Autodesk Inventor part; units mm, degrees
ref_plane "YZ Plane" through (0, 0, 0) normal (1, 0, 0) x (0, 1, 0)
ref_plane "XZ Plane" through (0, 0, 0) normal (0, 1, 0) x (-1, 0, 0)
ref_plane "XY Plane" through (0, 0, 0) normal (0, 0, 1) x (1, 0, 0)
sketch "스케치1" plane through (0, 0, 0) normal (0, 1, 0) x (-1, 0, 0)
  line L0 (-30, 30) -> (30, 30)
  line L1 (30, 30) -> (30, -30)
  line L2 (30, -30) -> (-30, -30)
  line L3 (-30, -30) -> (-30, 30)
  line L4 (-30, 30) -> (30, -30) construction
  line L5 (30, 30) -> (-30, -30) construction
  line L6 (-32.4, 32.4) -> (32.4, 32.4)
  line L7 (32.4, 32.4) -> (32.4, -32.4)
  line L8 (32.4, -32.4) -> (-32.4, -32.4)
  line L9 (-32.4, -32.4) -> (-32.4, 32.4)
  line L10 (-32.4, 32.4) -> (32.4, -32.4) construction
  line L11 (32.4, 32.4) -> (-32.4, -32.4) construction
  point P0 (0, 0)
  dimension "d45" = 60
  dimension "d46" = 60
  dimension "d47" = 2.4
extrude "돌출7" add sketch "스케치1" along normal blind 5 contours L0 L1 L2 L3 | L6 L7 L8 L9
sketch "스케치7" plane through (0, 5, 0) normal (0, 1, 0) x (1, 0, 0)
  line L0 (-30, -30) -> (30, -30)
  line L1 (30, -30) -> (30, 30)
  line L2 (30, 30) -> (-30, 30)
  line L3 (-30, 30) -> (-30, -30)
  line L4 (-30, -30) -> (30, 30) construction
  line L5 (30, -30) -> (-30, 30) construction
  line L6 (31.6, -31.6) -> (-31.6, -31.6)
  line L7 (-31.6, -31.6) -> (-31.6, 31.6)
  line L8 (-31.6, 31.6) -> (31.6, 31.6)
  line L9 (31.6, 31.6) -> (31.6, -31.6)
  line L10 (31.6, -31.6) -> (-31.6, 31.6) construction
  line L11 (-31.6, -31.6) -> (31.6, 31.6) construction
  point P0 (0, 0)
  dimension "d50" = 60
  dimension "d51" = 60
  dimension "d52" = 1.6
extrude "돌출8" cut sketch "스케치7" against normal blind 1.6
sketch "스케치8" plane through (0, 0, 0) normal (0, -1, 0) x (1, 0, 0)
  line L0 (-20, -2.5) -> (-10, -2.5)
  line L1 (-10, -2.5) -> (-10, 2.5)
  line L2 (-10, 2.5) -> (-20, 2.5)
  line L3 (-20, 2.5) -> (-20, -2.5)
  line L4 (-20, -2.5) -> (-10, 2.5) construction
  line L5 (-10, -2.5) -> (-20, 2.5) construction
  line L6 (10, -2.5) -> (20, -2.5)
  line L7 (20, -2.5) -> (20, 2.5)
  line L8 (20, 2.5) -> (10, 2.5)
  line L9 (10, 2.5) -> (10, -2.5)
  line L10 (10, -2.5) -> (20, 2.5) construction
  line L11 (20, -2.5) -> (10, 2.5) construction
  line L12 (32.4, 32.4) -> (32.4, -32.4)
  line L13 (32.4, 0) -> (20, 0)
  line L14 (-20, 0) -> (-32.4, 0)
  line L15 (-32.4, -32.4) -> (-32.4, 32.4)
  point P0 (0, 0)
  point P1 (-15, 0)
  point P2 (15, 0)
  dimension "d55" = 10
  dimension "d56" = 5
  dimension "d57" = 20
  dimension "d58" = 10
  dimension "d61" = 12.4
extrude "돌출9" add sketch "스케치8" along normal blind 10
sketch "스케치9" plane through (-10, 0, -2.5) normal (0, 0, -1) x (-1, 0, 0)
  line L0 (10, -10) -> (0, -10)
  circle A0 centre (5, -10) radius 5
  line L1 (-20, -10) -> (-30, -10)
  circle A1 centre (-25, -10) radius 5
  point P0 (-10, 0)
  dimension "d64" = 10
  dimension "d65" = 10
extrude "돌출10" add sketch "스케치9" against normal blind 5
sketch "스케치10" plane through (-10, 0, -2.5) normal (0, 0, -1) x (-1, 0, 0)
  arc A0 (0, -10) -> (10, -10) centre (5, -10) ccw
  circle A1 centre (5, -10) radius 1.25
  arc A2 (-30, -10) -> (-20, -10) centre (-25, -10) ccw
  circle A3 centre (-25, -10) radius 1.25
  point P0 (-10, 0)
  dimension "d68" = 2.5
  dimension "d69" = 2.5
extrude "돌출11" cut sketch "스케치10" against normal blind 5
sketch "스케치11" plane through (0, 0, 0) normal (0, -1, 0) x (1, 0, 0)
  circle A0 centre (0, 19.821) radius 1.25
  line L0 (-20, 2.5) -> (-10, 2.5)
  point P0 (0, 0)
  dimension "d72" = 2.5
  dimension "d73" = 17.321
extrude "돌출12" cut sketch "스케치11" against normal blind 5
properties part number "사각형 OV-PAM 5패턴 상단"
The model under review builds one solid part; all positions refer to its coordinate system, in mm. A direction names the side the tool comes from. Round coordinates to 2 decimals unless told otherwise and drop trailing zeros. Loops run counter-clockwise (first coordinate to the right, second up) from the corner with the lowest first, then second, coordinate; pieces in that order, holes last. Notation, with made-up numbers: M 76.25,39 L 109.25,39 A22 ccw 109.25,57 Z; hole C -32,-18 d11. An arc over 180 degrees is marked long. Write item = value, one per line.
Item 1: Take a section at B-B on z = 1.5. Write out the cut boundary in (x, y).
Return value:
outline = M -32.4,0 L -20,0 L -20,-10 A5 ccw -10,-10 L -10,0 L 10,0 L 10,-10 A5 ccw 20,-10 L 20,0 L 32.4,0 L 32.4,5 L 31.6,5 L 31.6,3.4 L 30,3.4 L 30,5 L -30,5 L -30,3.4 L -31.6,3.4 L -31.6,5 L -32.4,5 Z; hole C -15,-10 d2.5; hole C 15,-10 d2.5
Item 2: Take a section at D-D on x = 9. Write out the cut boundary in (y, z).
Return value:
outline = M 0,-32.4 L 5,-32.4 L 5,-31.6 L 3.4,-31.6 L 3.4,-30 L 5,-30 L 5,30 L 3.4,30 L 3.4,31.6 L 5,31.6 L 5,32.4 L 0,32.4 Z
Item 3: Take a section at C-C on x = -15. Write out the cut boundary in (y, z).
Return value:
outline = M -15,-2.5 L -11.25,-2.5 L -11.25,2.5 L -15,2.5 Z; M -8.75,-2.5 L 0,-2.5 L 0,-32.4 L 5,-32.4 L 5,-31.6 L 3.4,-31.6 L 3.4,-30 L 5,-30 L 5,30 L 3.4,30 L 3.4,31.6 L 5,31.6 L 5,32.4 L 0,32.4 L 0,2.5 L -8.75,2.5 Z
Item 4: Machinability: for faces 1 (the flat face through (-15, -7, -2.5)), 2 (the flat face through (30, 4, 0)), 3 (the flat face through (-10, -5, 0)), 4 (the flat face through (15, -7, 2.5)), which of the approach directions +Z, -Z, +X, -X, +Y, -Y give a long, thin tool a straight path to every point of the face, cutting with its end or side? Answer none if there is none.
Return value:
face_1 = -Z, +X, -X, -Y
face_2 = +Y
face_3 = +Z, -Z, -Y
face_4 = +Z, +X, -X, -Y
Item 5: Insertion check: P1, Ø2.5, axis at y = -4, z = 1, coming from the -X side; P2, Ø2, axis at x = -15, y = -10, coming from the -Z side; P3, Ø5, axis at x = 16.5, y = -11, coming from the -Z side; P4, Ø4, axis at y = -6, z = 1, coming from the +X side. Each pin has a flat end and moves straight along its axis. Give the tip position at first contact, or say it passes through.
Return value:
P1 = -20
P2 = through
P3 = -2.5
P4 = 20
Item 6: The part is to be moulded in two halves that separate along X. For faces 5 (the flat face through (0, 4, -31.6)), 6 (the flat face through (-32.4, 2, 0)), 7 (the flat face through (15, -7, -2.5)), say which applies: released by +X, released by -X, zero draft, split by the parting line, or undercut.
Return value:
face_5 = undercut
face_6 = released by -X
face_7 = zero draft
Item 7: For line 1 (Z direction, x = 0, y = 3.6); line 2 (X direction, y = 4, z = 17); line 3 (Y direction, x = 15, z = 1.2), list the stretches that pass through material, from the lowest coordinate up. Write a range as [from, to].
Return value:
line_1 = [-32.4, -31.6], [-30, 18.57], [21.07, 30], [31.6, 32.4]
line_2 = [-32.4, -31.6], [-30, 30], [31.6, 32.4]
line_3 = [-15, -11.25], [-8.75, 5]
Item 8: Take a section at A-A on y = -6.5. Write out the cut boundary in (x, z).
Return value:
outline = M -20,-2.5 L -10,-2.5 L -10,2.5 L -20,2.5 Z; M 10,-2.5 L 20,-2.5 L 20,2.5 L 10,2.5 Z
